Read the model definition and answer for the solid it produces. Units are mm, in the model's axes. Face numbers are marked on the shaded views. Give positions to 0.01 mm unless a question says otherwise; leave off trailing zeros. Write each loop counter-clockwise with the first axis right and the second up, starting at its lowest first coordinate (ties: lowest second). Pieces come first, ordered by that corner, then holes. Notation, with made-up numbers: (70.25, 36.5) -> (79.25, 36.5) arc R28 cw to (79.25, 70.5) -> close; hole circle Ø1 at (47, 16.25). An arc over 180 degrees is marked (long way). Answer as CSV lines item,"result". Start each with the question number.
1. The part is cut by section B-B, the plane x = 0. Determine the outline of the cut face in (y, z), and give its area (3 significant figures).
2. For a pull along X with two mould halves and no side action, classify the marked faces 1 and 2 as pulls with the +X half, pulls with the -X half, needs draft (parallel to the pull), parting line crosses it, or undercut.
3. The part is cut by section C-C, the plane z = -32. Determine the outline of the cut face in (x, y).
4. Given pin 1 (0.8 mm diameter, centred on x = 5, y = 1.5, fed in from -Z); pin 2 (0.8 mm diameter, centred on y = 2, z = -25, fed in from +X); pin 3 (0.8 mm diameter, centred on x = 0.5, y = 1.5, fed in from +Z); pin 4 (3 mm diameter, centred on y = 2.5, z = 14.5, fed in from +X), each flat-ended and moving along its own axis, determine where each tip first touches the part or whether it passes through.
5. Find the intervals of material crossed by line 1 (Z direction, x = 2, y = 4.5); line 2 (X direction, y = 1.75, z = -65.5); line 3 (X direction, y = 2, z = -71.5), in increasing order.
6. The part is cut by section A-A, the plane y = 5.25. Determine the outline of the cut face in (x, z), and give its area (3 significant figures).
7. The part is cut by section D-D, the plane x = -38.5. Determine the outline of the cut face in (y, z).
from build123d import *

# Parameters (mm, degrees)
SKETCH1_W           = 25.4
SKETCH1_H           = 25.4
BOSS_EXTRUDE1_DEPTH = 6.35
SKETCH2_R           = 6.35
SKETCH2_R_2         = 6.382099354
CUT_EXTRUDE1_DEPTH  = 108.784518461
SKETCH3_W           = 24.960329338
SKETCH3_H           = 23.230097692
CUT_EXTRUDE2_DEPTH  = 2.54


with BuildPart() as part:
    # Sketch1 → Boss-Extrude1 (new body)
    with BuildSketch(Plane(origin=(0, 0, 0), x_dir=(1, 0, 0), z_dir=(0, 1, 0))):
        with BuildLine():
            Line((12.7, 36.061556053), (12.7, 74.161556053))
            ThreePointArc((12.7, 74.161556053), (0, 86.861556053), (-12.7, 74.161556053))
            Line((-12.7, 74.161556053), (-12.7, 36.061556053))
            Line((-12.7, 36.061556053), (12.7, 36.061556053))
        make_face()
        with BuildLine():
            Line((50.8, 36.061556053), (12.7, 36.061556053))
            Line((12.7, 36.061556053), (12.7, 10.661556053))
            Line((12.7, 10.661556053), (50.8, 10.661556053))
            ThreePointArc((50.8, 10.661556053), (63.5, 23.361556053), (50.8, 36.061556053))
        make_face()
        with BuildLine():
            Line((12.7, -27.438443947), (12.7, 10.661556053))
            Line((12.7, 10.661556053), (-12.7, 10.661556053))
            Line((-12.7, 10.661556053), (-12.7, -27.438443947))
            ThreePointArc((-12.7, -27.438443947), (0, -40.138443947), (12.7, -27.438443947))
        make_face()
        with BuildLine():
            Line((-12.7, 10.661556053), (-12.7, 36.061556053))
            Line((-12.7, 36.061556053), (-50.8, 36.061556053))
            ThreePointArc((-50.8, 36.061556053), (-63.5, 23.361556053), (-50.8, 10.661556053))
            Line((-50.8, 10.661556053), (-12.7, 10.661556053))
        make_face()
        with Locations((0, 23.361556053)):
            Rectangle(SKETCH1_W, SKETCH1_H)
    extrude(amount=BOSS_EXTRUDE1_DEPTH)

    # Sketch2 → Cut-Extrude1 (cut, through all)
    with BuildSketch(Plane(origin=(0, 6.35, 0), x_dir=(1, 0, 0), z_dir=(0, 1, 0))):
        with Locations(Location((0, 74.161556053, 0), (0, 0, 270))):
            Circle(SKETCH2_R)
        with Locations(Location((-50.8, 23.361556053, 0), (0, 0, 270))):
            Circle(SKETCH2_R)
        with Locations(Location((0, -27.438443947, 0), (0, 0, 270))):
            Circle(SKETCH2_R_2)
        with Locations(Location((50.8, 23.361556053, 0), (0, 0, 270))):
            Circle(SKETCH2_R)
    extrude(amount=-CUT_EXTRUDE1_DEPTH, mode=Mode.SUBTRACT)

    # Sketch3 → Cut-Extrude2 (cut)
    with BuildSketch(Plane(origin=(0, 0, 0), x_dir=(1, 0, 0), z_dir=(0, 1, 0))):
        with Locations((-0.219835331, 23.57664955)):
            Rectangle(SKETCH3_W, SKETCH3_H)
    extrude(amount=CUT_EXTRUDE2_DEPTH, mode=Mode.SUBTRACT)


solid = part.part
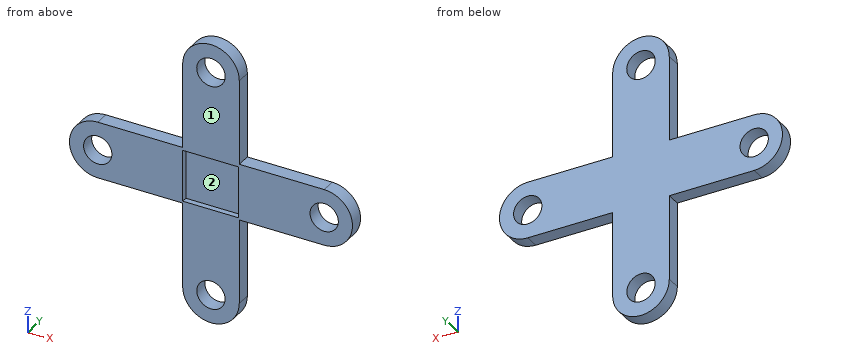
Results found:
1,outline,"(0, -86.86) -> (6.35, -86.86) -> (6.35, -80.51) -> (0, -80.51) -> close; (0, -67.81) -> (6.35, -67.81) -> (6.35, 21.06) -> (0, 21.06) -> (0, -11.96) -> (2.54, -11.96) -> (2.54, -35.19) -> (0, -35.19) -> close; (0, 33.82) -> (6.35, 33.82) -> (6.35, 40.14) -> (0, 40.14) -> close"
1,area,"586 mm²"
2,face 1,"needs draft"
2,face 2,"undercut"
3,outline,"(-60.11, 0) -> (-12.7, 0) -> (-12.7, 2.54) -> (12.26, 2.54) -> (12.26, 0) -> (60.11, 0) -> (60.11, 6.35) -> (-60.11, 6.35) -> close"
4,pin 1,"stops at z = -86"
4,pin 2,"stops at x = 63.44"
4,pin 3,"stops at z = 40.14"
4,pin 4,"stops at x = 12.7"
5,line 1,"z = -86.7 to -80.19, -68.13 to 21.38, 33.5 to 39.98"
5,line 2,"x = -12.7 to 12.7"
5,line 3,"x = -12.7 to -5.77, 5.77 to 12.7"
6,outline,"(-50.8, -36.06) -> (-12.7, -36.06) -> (-12.7, -74.16) arc R12.7 ccw to (12.7, -74.16) -> (12.7, -36.06) -> (50.8, -36.06) arc R12.7 ccw to (50.8, -10.66) -> (12.7, -10.66) -> (12.7, 27.44) arc R12.7 ccw to (-12.7, 27.44) -> (-12.7, -10.66) -> (-50.8, -10.66) arc R12.7 ccw to start; hole circle Ø12.7 at (-50.8, -23.36); hole circle Ø12.76 at (0, 27.44); hole circle Ø12.7 at (0, -74.16); hole circle Ø12.7 at (50.8, -23.36)"
6,area,"5,020 mm²"
7,outline,"(0, -36.06) -> (6.35, -36.06) -> (6.35, -10.66) -> (0, -10.66) -> close"
